Could you check a few things on this model? Use its own coordinates, in mm. A direction names the side the tool comes from. Round coordinates to 2 decimals unless told otherwise and drop trailing zeros. Order: outer loops, then holes, each group sorted by start corner. A loop starts at its lowest first (then second) coordinate and runs counter-clockwise, first axis right, second up. Notation, with made-up numbers: (-6, 86.25) - (-1, 86.25) arc R9 cw to (-1, 94.25) - close; hole circle Ø4 at (53, -28.5). An arc over 180 degrees is marked (long way). Use one line per item in the form item = value.
from build123d import *

# Parameters (mm, degrees)
SKETCH_1_W      = 2.5
SKETCH_1_H      = 4
EXTRUDE_1_DEPTH = 8
SKETCH_2_W      = 15
SKETCH_2_H      = 20
EXTRUDE_2_DEPTH = 2


with BuildPart() as part:
    # 草图1 → 凸台-拉伸1 (new body)
    with BuildSketch(Plane(origin=(0, 0, 0), x_dir=(1, 0, 0), z_dir=(0, 1, 0))):
        with Locations((1.25, 2)):
            Rectangle(SKETCH_1_W, SKETCH_1_H)
    extrude(amount=EXTRUDE_1_DEPTH)

    # 草图2 → 凸台-拉伸2 (add)
    with BuildSketch(Plane.XZ):
        with Locations((-5, 6)):
            Rectangle(SKETCH_2_W, SKETCH_2_H)
    extrude(amount=EXTRUDE_2_DEPTH)


solid = part.part
Item 1: Imagine slicing it at D-D on z = 4.5. Please give me the cut outline in (x, y), plus the area to 3 significant figures.
Found:
outline = (-12.5, -2) - (2.5, -2) - (2.5, 0) - (-12.5, 0) - close
area = 30.0 mm2
Item 2: Imagine slicing it at A-A on z = -2.5. Please give me the cut outline in (x, y), plus the area to 3 significant figures.
Found:
outline = (-12.5, -2) - (2.5, -2) - (2.5, 8) - (0, 8) - (0, 0) - (-12.5, 0) - close
area = 50.0 mm2
Item 3: I need wall thicknesses on L1, parallel to Y at x = -1.75, z = 10; L2, parallel to Z at x = 1, y = 7.5. Which ranges of each line are inside material? Lowest first, please.
Found:
L1 = -2 to 0
L2 = -4 to 0
Item 4: Imagine slicing it at C-C on y = 1.25. Please give me the cut outline in (x, z).
Found:
outline = (0, -4) - (2.5, -4) - (2.5, 0) - (0, 0) - close
Item 5: For faces 1 (the face through (1, 4, 0)), 2 (the face through (0, 4, -2)), 3 (the face through (-2.8, -0.3, -4)), which set-ups out of +Z, -Z, +X, -X, +Y, -Y let a thin tool reach every point of the face, with its end or its side?
Found:
face_1 = +Z, +X, -X, +Y
face_2 = +Z, -Z, -X, +Y
face_3 = -Z, +X, -X, +Y, -Y
Item 6: Imagine slicing it at B-B on x = 1. Please give me the cut outline in (y, z).
Found:
outline = (-2, -4) - (8, -4) - (8, 0) - (0, 0) - (0, 16) - (-2, 16) - close
Item 7: Will these pins go through, and if not, where does the flat tip stop? P1, Ø5, axis at y = 5.5, z = 3.5, coming from the +X side; P2, Ø2, axis at y = 2, z = -1, coming from the -X side; P3, Ø3, axis at x = 0.5, y = 2.5, coming from the +Z side.
Found:
P1 = through
P2 = 0
P3 = 0
